```python
from build123d import *

# Parameters (mm, degrees)
SKETCH_1_W             = 30
SKETCH_1_H             = 32.3
EXTRUDE_417_DEPTH      = 4
EXTRUDE_710_DEPTH      = 12
SKETCH_4_R             = 1.5
CUT_EXTRUDE_1014_DEPTH = 36.296210845
CHAMFER_1_SIZE         = 1.5
SKETCH_3_R             = 0.75
CUT_EXTRUDE_1313_DEPTH = 10
SKETCH_5_W             = 2.5
SKETCH_5_H             = 8.5
CUT_EXTRUDE_1575_DEPTH = 4.15
FILLET_1_R             = 2
CUT_EXTRUDE_2459_REACH = 29.236
SKETCH_7_R             = 1.35
CUT_EXTRUDE_3094_DEPTH = 2.15
FILLET_2_R             = 3


with BuildPart() as part:
    # Эскиз1 → Extrude 417 (new body)
    with BuildSketch(Plane.XY):
        Rectangle(SKETCH_1_W, SKETCH_1_H)
    extrude(amount=EXTRUDE_417_DEPTH)

    # Эскиз2 → Extrude 710 (add)
    with BuildSketch(Plane.XY.offset(4)):
        Polygon((8, 16.15), (-15, 16.15), (-15, -16.15), (8, -16.15), (8, -12), (-12, -12), (-12, 12), (8, 12), align=None)
    extrude(amount=EXTRUDE_710_DEPTH)

    # Эскиз4 → Cut-Extrude 1014 (cut, through all)
    with BuildSketch(Plane(origin=(-12, 0, 0), x_dir=(0, 0, -1), z_dir=(1, 0, 0))):
        with Locations(Location((-10, -5.77, 0), (0, 0, 90))):
            Circle(SKETCH_4_R)
    extrude(amount=-CUT_EXTRUDE_1014_DEPTH, mode=Mode.SUBTRACT)

    # Фаска1
    chamfer_1_edges = [part.edges().sort_by_distance(p)[0] for p in [
        (-12, -7.27, 10),
    ]]
    chamfer(chamfer_1_edges, length=CHAMFER_1_SIZE)

    # Эскиз3 → Cut-Extrude 1313 (cut)
    with BuildSketch(Plane(origin=(8, 0, 0), x_dir=(0, 0, -1), z_dir=(1, 0, 0))):
        with Locations((-10, 14.32)):
            Circle(SKETCH_3_R)
    cut_extrude_1313 = extrude(amount=-CUT_EXTRUDE_1313_DEPTH, mode=Mode.SUBTRACT)

    # Зеркальное отражение2: Cut-Extrude 1313 across plane
    add(cut_extrude_1313.mirror(Plane.ZX), mode=Mode.SUBTRACT)

    # Эскиз5 → Cut-Extrude 1575 (cut)
    with BuildSketch(Plane.XZ.offset(16.15)):
        with Locations((-7.35, 11.75)):
            Rectangle(SKETCH_5_W, SKETCH_5_H)
    extrude(amount=-CUT_EXTRUDE_1575_DEPTH, mode=Mode.SUBTRACT)

    # Скругление1
    fillet_1_edges = [part.edges().sort_by_distance(p)[0] for p in [
        (15, -16.15, 2),
        (-15, -16.15, 8),
        (-15, 16.15, 8),
        (15, 16.15, 2),
    ]]
    fillet(fillet_1_edges, radius=FILLET_1_R)

    # Эскиз7 → Cut-Extrude 2459 (cut, up to next)
    with BuildSketch(Plane(origin=(0, 0, 0), x_dir=(-1, 0, 0), z_dir=(0, 0, -1)), mode=Mode.PRIVATE) as cut_extrude_2459_sk1:
        with Locations((10.5, 6.75)):
            Circle(SKETCH_7_R)
    cut_extrude_2459_tool1 = extrude(cut_extrude_2459_sk1.sketch, amount=-CUT_EXTRUDE_2459_REACH, mode=Mode.PRIVATE) & part.part
    # Эскиз7 → Cut-Extrude 2459 (cut, up to next)
    with BuildSketch(Plane(origin=(0, 0, 0), x_dir=(-1, 0, 0), z_dir=(0, 0, -1)), mode=Mode.PRIVATE) as cut_extrude_2459_sk2:
        with Locations((-10.5, 6.75)):
            Circle(SKETCH_7_R)
    cut_extrude_2459_tool2 = extrude(cut_extrude_2459_sk2.sketch, amount=-CUT_EXTRUDE_2459_REACH, mode=Mode.PRIVATE) & part.part
    # Эскиз7 → Cut-Extrude 2459 (cut, up to next)
    with BuildSketch(Plane(origin=(0, 0, 0), x_dir=(-1, 0, 0), z_dir=(0, 0, -1)), mode=Mode.PRIVATE) as cut_extrude_2459_sk3:
        with Locations((-10.5, -6.75)):
            Circle(SKETCH_7_R)
    cut_extrude_2459_tool3 = extrude(cut_extrude_2459_sk3.sketch, amount=-CUT_EXTRUDE_2459_REACH, mode=Mode.PRIVATE) & part.part
    # Эскиз7 → Cut-Extrude 2459 (cut, up to next)
    with BuildSketch(Plane(origin=(0, 0, 0), x_dir=(-1, 0, 0), z_dir=(0, 0, -1)), mode=Mode.PRIVATE) as cut_extrude_2459_sk4:
        with Locations((10.5, -6.75)):
            Circle(SKETCH_7_R)
    cut_extrude_2459_tool4 = extrude(cut_extrude_2459_sk4.sketch, amount=-CUT_EXTRUDE_2459_REACH, mode=Mode.PRIVATE) & part.part
    add(cut_extrude_2459_tool1.solids().sort_by_distance((-10.5, 6.75, 0))[0], mode=Mode.SUBTRACT)
    add(cut_extrude_2459_tool2.solids().sort_by_distance((10.5, 6.75, 0))[0], mode=Mode.SUBTRACT)
    add(cut_extrude_2459_tool3.solids().sort_by_distance((10.5, -6.75, 0))[0], mode=Mode.SUBTRACT)
    add(cut_extrude_2459_tool4.solids().sort_by_distance((-10.5, -6.75, 0))[0], mode=Mode.SUBTRACT)

    # Эскиз8 → Cut-Extrude 3094 (cut)
    with BuildSketch(Plane.XY.offset(4)):
        Polygon((10.5, 9.809956427), (7.85, 8.279978213), (7.85, 5.220021787), (10.5, 3.690043573), (13.15, 5.220021787), (13.15, 8.279978213), align=None)
        Polygon((-13.15, 8.279978213), (-10.5, 9.809956427), (-7.85, 8.279978213), (-7.85, 5.220021787), (-10.5, 3.690043573), (-13.15, 5.220021787), align=None)
        Polygon((-10.5, -9.809956427), (-7.85, -8.279978213), (-7.85, -5.220021787), (-10.5, -3.690043573), (-13.15, -5.220021787), (-13.15, -8.279978213), align=None)
        Polygon((13.15, -8.279978213), (10.5, -9.809956427), (7.85, -8.279978213), (7.85, -5.220021787), (10.5, -3.690043573), (13.15, -5.220021787), align=None)
    extrude(amount=-CUT_EXTRUDE_3094_DEPTH, mode=Mode.SUBTRACT)

    # Скругление2
    # the kernel refuses this fillet: 3 mm, written as the material it takes off along each edge
    with BuildSketch(Plane(origin=(20.5, 16.15, 0), x_dir=(0, -1, 0), z_dir=(-1, 0, 0))) as fillet_2_piece_1:
        with BuildLine():
            CenterArc((FILLET_2_R, FILLET_2_R), FILLET_2_R, 180, 90)
            Line((0, FILLET_2_R), (0, 0))
            Line((0, 0), (FILLET_2_R, 0))
        make_face()
    extrude(amount=41, mode=Mode.SUBTRACT)


solid = part.part
```
Work out the finished part from the listing and answer in its coordinate system (mm). A direction names the side the tool comes from. Round coordinates to 2 decimals unless told otherwise and drop trailing zeros. Loops run counter-clockwise (first coordinate to the right, second up) from the corner with the lowest first, then second, coordinate; pieces in that order, holes last. Notation, with made-up numbers: M -39.75,-35 L 6.25,-35 A19 cw 6.25,-26 Z; hole C 89,42 d6. An arc over 180 degrees is marked long. One line per question, with ' | ' between items.
Q1. Each of these flat-tipped pins is pushed along its axis until it touches: pin 1 Ø1 at (x, y) = (1.5, 1) entering from +Z; pin 2 Ø6 at (x, y) = (5.5, 11) entering from -Z; pin 3 Ø4.5 at (y, z) = (-14.5, 11) entering from +X; pin 4 Ø4 at (y, z) = (4, 12.5) entering from +X. Where does it stop, or does it pass through?
Conclusion:
pin 1: stops at z = 4 | pin 2: stops at z = 0 | pin 3: stops at x = 8 | pin 4: stops at x = -12
Q2. The mould has two halves that part along X. Classify faces 4 (the cylindrical face through (-14.4, 15.58, 8.2)), 5 (the flat face through (-7.85, 7, 3)), 6 (the cylindrical face through (14.626, 15.315, 2.538)), 7 (the flat face through (-9.156, -4.466, 2.94)): +X half, -X half, draft (parallel to the pull), parting line (faces both ways), or undercut.
Conclusion:
face 4: -X half | face 5: undercut | face 6: +X half | face 7: undercut
Q3. Find section A-A, the plane z = 14.5. Give the vertices of the cut face in (x, y).
Conclusion:
outline: M -15,-14.15 A2 ccw -13,-16.15 L -8.6,-16.15 L -8.6,-12 L -12,-12 L -12,12 L 8,12 L 8,16.15 L -13,16.15 A2 ccw -15,14.15 Z; M -6.1,-16.15 L 8,-16.15 L 8,-12 L -6.1,-12 Z
Q4. Find section B-B, the plane x = -1.5. Give the vertices of the cut face in (y, z).
Conclusion:
outline: M -16.15,0 L 13.15,0 A3 ccw 16.15,3 L 16.15,16 L 12,16 L 12,4 L -12,4 L -12,16 L -16.15,16 Z; hole C -14.32,10 d1.5; hole C 14.32,10 d1.5
Q5. A tool of negligible diameter and unlimited length cuts with its end or side. For faces 1 (the flat face through (-9, 6, 1.85)), 2 (the cylindrical face through (3.07, -13.588, 10.163)), 3 (the flat face through (7.85, 7, 3)), from which of +Z, -Z, +X, -X, +Y, -Y can it reach the whole face along a straight path? Write none if from no direction.
Conclusion:
face 1: none | face 2: +X | face 3: +Z
Q6. Consider line 1 along Y through (x, z) = (1, 10); line 2 along X through (y, z) = (-6, 3); line 3 along Y through (x, z) = (-5, 8.75). Determine where each line is inside the solid, lowest interval first. Write a range as from..to.
Conclusion:
line 1: y = -16.15..-15.07, -13.57..-12, 12..13.57, 15.07..16.15 | line 2: x = -15..-13.15, -7.85..7.85, 13.15..15 | line 3: y = -16.15..-12, 12..16.15
Q7. Find section D-D, the plane z = 6.5. Give the vertices of the cut face in (x, y).
Conclusion:
outline: M -15,-14.15 A2 ccw -13,-16.15 L 8,-16.15 L 8,-12 L -12,-12 L -12,12 L 8,12 L 8,16.15 L -13,16.15 A2 ccw -15,14.15 Z
Q8. Find section C-C, the plane y = 6.75. Give the vertices of the cut face in (x, z), then the cut area to 3 significant figures.
Conclusion:
outline: M -15,0 L -11.85,0 L -11.85,1.85 L -13.15,1.85 L -13.15,4 L -12,4 L -12,16 L -15,16 Z; M -9.15,0 L 9.15,0 L 9.15,1.85 L 7.85,1.85 L 7.85,4 L -7.85,4 L -7.85,1.85 L -9.15,1.85 Z; M 11.85,0 L 15,0 L 15,4 L 13.15,4 L 13.15,1.85 L 11.85,1.85 Z | area: 123 mm2
